Autodesk Inventor part; units mm, degrees
ref_plane "YZ Plane" through (0, 0, 0) normal (1, 0, 0) x (0, 1, 0)
ref_plane "XZ Plane" through (0, 0, 0) normal (0, 1, 0) x (-1, 0, 0)
ref_plane "XY Plane" through (0, 0, 0) normal (0, 0, 1) x (1, 0, 0)
sketch "Boceto1" plane through (0, 0, 0) normal (0, 0, 1) x (1, 0, 0)
  circle A0 centre (0, 0) radius 8.9
  line L0 (6.2933, -6.2933) -> (-6.2933, -6.2933)
  line L1 (-6.2933, -6.2933) -> (-6.2933, 6.2933)
  line L2 (-6.2933, 6.2933) -> (6.2933, 6.2933)
  line L3 (6.2933, 6.2933) -> (6.2933, -6.2933)
  dimension "d0" = 17.8
  dimension "d1" = 12.5865
  dimension "d2" = 12.5865
extrude "Extrusión1" add sketch "Boceto1" along normal blind 32 contours L3 L0 L1 L2
sketch "Boceto3" plane through (0, 0, 0) normal (0, 0, -1) x (-1, 0, 0)
  circle A0 centre (0, 0) radius 2
  dimension "d25" = 4
extrude "Extrusión3" cut sketch "Boceto3" against normal blind 20
sketch "Boceto4" plane through (0, 0, 0) normal (0, 1, 0) x (-1, 0, 0)
  line L0 (-6.2933, 0) -> (6.2933, 0)
  line L1 (-6.2933, 0) -> (6.2933, 0)
  line L2 (6.2933, 0) -> (6.2933, 2)
  line L3 (6.2933, 2) -> (-6.2933, 2)
  line L4 (-6.2933, 2) -> (-6.2933, 0)
  line L5 (-6.2933, 0) -> (-4.2933, 0)
  line L6 (-4.2933, 0) -> (-4.2933, 5)
  line L7 (-4.2933, 5) -> (-6.2933, 5)
  line L8 (-6.2933, 5) -> (-6.2933, 0)
  line L9 (6.2933, 0) -> (4.2933, 0)
  line L10 (4.2933, 0) -> (4.2933, 5)
  line L11 (4.2933, 5) -> (6.2933, 5)
  line L12 (6.2933, 5) -> (6.2933, 0)
  line L13 (-6.2933, 5) -> (6.2933, 5)
  line L14 (6.2933, 5) -> (6.2933, 7)
  line L15 (6.2933, 7) -> (-6.2933, 7)
  line L16 (-6.2933, 7) -> (-6.2933, 5)
  line L17 (0, 7) -> (6.2933, 7)
  line L18 (0, 7) -> (-6.2933, 7)
  line L19 (3.1484, 5.1198) -> (-3.993, 16.4674)
  line L20 (-4.8411, 17.815) -> (-3.9947, 18.3476)
  line L21 (4.8411, 6.185) -> (3.1484, 5.1198)
  line L22 (-5.1073, 15.7625) -> (-3.4147, 14.697)
  line L23 (3.9942, 27.532) -> (-0.0773, 34)
  line L24 (-3.4155, 39.303) -> (-5.1081, 38.2376)
  line L25 (-6.2933, 32) -> (6.2933, 32)
  line L26 (-6.2933, 32) -> (6.2933, 32)
  line L27 (6.2933, 32) -> (6.2933, 34)
  line L28 (6.2933, 34) -> (-6.2933, 34)
  line L29 (-6.2933, 34) -> (-6.2933, 32)
  line L30 (-1.6298, 16.4672) -> (4.8411, 6.185)
  line L31 (-1.6297, 17.5326) -> (3.9942, 26.4665)
  line L32 (-2.4406, 34) -> (1.6309, 27.532)
  line L33 (-2.4406, 34) -> (-0.0773, 34)
  line L34 (1.6309, 26.4665) -> (-3.9929, 17.5327)
  line L35 (0, 0) -> (0, -2)
  arc A0 (-1.6297, 17.5326) -> (-1.6298, 16.4672) centre (-0.7834, 16.9999) ccw
  arc A1 (-3.9929, 17.5327) -> (-3.993, 16.4674) centre (-3.1466, 17) ccw
  arc A2 (1.6309, 26.4665) -> (1.6309, 27.532) centre (0.7846, 26.9993) ccw
  arc A3 (3.9942, 26.4665) -> (3.9942, 27.532) centre (3.1479, 26.9993) ccw
  line L36 (-3.1484, 5.1198) -> (3.993, 16.4674)
  line L37 (-4.8411, 6.185) -> (-3.1484, 5.1198)
  line L38 (-3.9942, 27.532) -> (0.0773, 34)
  line L39 (1.6298, 16.4672) -> (-4.8411, 6.185)
  line L40 (1.6297, 17.5326) -> (-3.9942, 26.4665)
  line L41 (2.4406, 34) -> (-1.6309, 27.532)
  line L42 (2.4406, 34) -> (0.0773, 34)
  line L43 (-1.6309, 26.4665) -> (3.9929, 17.5327)
  arc A4 (1.6298, 16.4672) -> (1.6297, 17.5326) centre (0.7834, 16.9999) ccw
  arc A5 (3.993, 16.4674) -> (3.9929, 17.5327) centre (3.1466, 17) ccw
  arc A6 (-1.6309, 27.532) -> (-1.6309, 26.4665) centre (-0.7846, 26.9993) ccw
  arc A7 (-3.9942, 27.532) -> (-3.9942, 26.4665) centre (-3.1479, 26.9993) ccw
  point P0 (3.1466, 7)
  point P1 (-3.1466, 7)
  point P2 (0.0009, 22)
  point P3 (0, 32)
  point P4 (3.4147, 14.697)
  point P5 (-0.0009, 22)
  point P6 (3.9947, 18.3476)
  point P7 (-4.2933, 2)
  point P8 (4.2933, 2)
  point P9 (0, 10.1225)
  point P10 (1.9651, 7)
  point P11 (-1.9651, 7)
  point P12 (0, 13.8775)
  point P13 (0, 20.1215)
  point P14 (0, 30.1229)
  point P15 (0, 23.8757)
  point P16 (4.3282, 7)
  point P17 (1.1815, 12)
  point P18 (1.1816, 21.9986)
  point P19 (1.1816, 32)
  point P20 (-1.1816, 32)
  point P21 (-1.1816, 21.9986)
  point P22 (-1.1815, 12)
  point P23 (-4.3282, 7)
  dimension "d28" = 2
  dimension "d29" = 2
  dimension "d30" = 5
  dimension "d31" = 2
  dimension "d32" = 5
  dimension "d33" = 2
  dimension "d36" = 15
  dimension "d44" = 2
  dimension "d45" = 2
  dimension "d46" = 1
extrude "Extrusión4" cut sketch "Boceto4" against normal mid plane 100 contours L4 L3 L6 L0 | L6 L3 L10 L0 | L8 L7 L6 L3 | L16 L15 L39 L37 L36 L19 L21 L30 L14 L11 L13 L7 | L10 L3 L2 L0 | L10 L11 L12 L3 | L39 L19 L36 L15 | L15 L36 L37 L39 | L39 L30 L36 L19 | L19 A1 L34 L40 L31 A0 L30 L39 | L36 L30 L15 L19 | L39 A4 L40 L31 L43 A5 L36 L30 | L30 L21 L19 L15 | L40 A7 L38 L32 L41 A6 L43 L34 | L34 L43 L31 L40 | L34 A2 L32 L41 L23 A3 L31 L43 | L38 L23 L25 | L25 L29 L28 L32 | L25 L41 L32 | L32 L28 L23 L38 | L41 L28 L27 L25 | L23 L38 L28 L41 | L23 L28 L38 keep common part
extrude "Extrusión5" add sketch "Boceto4" along normal mid plane 12.5865 contours L38 L23 L25 | L25 L29 L28 L32 | L32 L28 L23 L38 | L41 L28 L27 L25 | L23 L38 L28 L41 | L23 L28 L38
properties part number "_3DPrint"
Geometry: final body of the model. Coordinates: model frame, mm. A direction names the side the tool comes from. Round coordinates to 2 decimals unless told otherwise and drop trailing zeros. Order: outer loops, then holes, each group sorted by start corner. A loop starts at its lowest first (then second) coordinate and runs counter-clockwise, first axis right, second up. Notation, with made-up numbers: (80.5, 46) -> (92.5, 46) arc R31 ccw to (92.5, 74) -> close; hole circle Ø10 at (-37.75, 53). An arc over 180 degrees is marked (long way). Use CSV: the item, a comma, the result in double quotes. Start each with the question number.
1) Material intervals for line 1 along Y through (x, z) = (0, 0.65); line 2 along Z through (x, y) = (5, 3.5); line 3 along Z through (x, y) = (0.5, -3.5), sorted ascending. Write a range as from..to.
2) First-contact query: pin 1 Ø0.6 at (x, y) = (1, 0.5) entering from -Z. Flat tip, straight axial feed; report the tip coordinate or a pass-through.
3) Section B-B (z = 8). Return the cut outline in (x, y), and give its area (3 significant figures).
4) Section D-D (y = 0). State how many separate pieces and enclosed holes the cut face has, and give its area (3 significant figures).
5) Section C-C (x = 2.5). Return the cut outline in (y, z), and give its area (3 significant figures).
6) Set-up query: faces 4 (the face through (-2.568, 0.088, 19.797)), 5 (the face through (1.783, 3.637, 17.008)), 6 (the face through (-1, 0, 20)), 7 (the face through (2.61, 0.09, 29.73)). Return all of +Z, -Z, +X, -X, +Y, -Y with unobstructed straight access to the full face (end or side cutting, diameter ignored); none if empty.
7) Draft query along Z for faces 1 (the face through (1, 0, 20)), 2 (the face through (0, -6.293, 33)), 3 (the face through (-2.73, 0.09, 9.54)). Return one class per face: +Z half, -Z half, draft (parallel to the pull), parting line (faces both ways), or undercut.
8) Section A-A (x = 4.75). Return the cut outline in (y, z), and give its area (3 significant figures).
Returned:
1,line 1,"y = -6.29..-2, 2..6.29"
1,line 2,"z = 0..7, 32..34"
1,line 3,"z = 0..2, 5..7, 9.33..14.67, 19.33..24.67, 29.33..34"
2,pin 1,"stops at z = 20"
3,outline,"(-3.7, -6.29) -> (-1.34, -6.29) -> (-1.34, -1.49) arc R2 cw to (-1.34, 1.49) -> (-1.34, 6.29) -> (-3.7, 6.29) -> close; (1.34, -6.29) -> (3.7, -6.29) -> (3.7, 6.29) -> (1.34, 6.29) -> (1.34, 1.49) arc R2 cw to (1.34, -1.49) -> close"
3,area,"56.7 mm²"
4,separate pieces,"3"
4,enclosed holes,"1"
4,area,"147 mm²"
5,outline,"(-6.29, 0) -> (6.29, 0) -> (6.29, 2) -> (-6.29, 2) -> close; (-6.29, 5) -> (6.29, 5) -> (6.29, 9.9) -> (-6.29, 9.9) -> close; (-6.29, 14.1) -> (6.29, 14.1) -> (6.29, 19.9) -> (-6.29, 19.9) -> close; (-6.29, 24.09) -> (6.29, 24.09) -> (6.29, 29.91) -> (-6.29, 29.91) -> close; (-6.29, 32) -> (6.29, 32) -> (6.29, 34) -> (-6.29, 34) -> close"
5,area,"258 mm²"
6,face 4,"-X, +Y, -Y"
6,face 5,"+Y, -Y"
6,face 6,"-Z"
6,face 7,"+X, +Y, -Y"
7,face 1,"-Z half"
7,face 2,"draft"
7,face 3,"undercut"
8,outline,"(-6.29, 0) -> (6.29, 0) -> (6.29, 7) -> (-6.29, 7) -> close; (-6.29, 32) -> (6.29, 32) -> (6.29, 34) -> (-6.29, 34) -> close"
8,area,"113 mm²"
